Job drawing, mm, ordinate dimensions from the low corner. One solid piece. Round coordinates to 2 decimals unless told otherwise and drop trailing zeros. Loops run counter-clockwise (first coordinate to the right, second up) from the corner with the lowest first, then second, coordinate; pieces in that order, holes last. Notation, with made-up numbers: M 22.5,83 L 43.5,83 A14 ccw 43.5,110 Z; hole C 31,14.5 d3. An arc over 180 degrees is marked long. Put each result on its own line as item: value. Start each with the question number.
1) Slice it at C-C on z = 20. Give the cut face in (x, y).
2) Slice it at A-A on z = 49. Give the cut face in (x, y), then the cut area to 3 significant figures.
3) Probe line 1 along Z through (x, y) = (50, 4.5); line 2 along Z through (x, y) = (27.5, 4.6). List the from-to ranges inside material, lowest first.
4) Slice it at D-D on x = 49. Give the cut face in (y, z).
5) Drop flat-ended pins along their axis: pin 1 Ø1.5 at (y, z) = (2, 45) entering from -X; pin 2 Ø1.5 at (x, y) = (34, 3.5) entering from -Z. Give the stop position or say it passes through.
6) Slice it at B-B on x = 31. Give the cut face in (y, z).
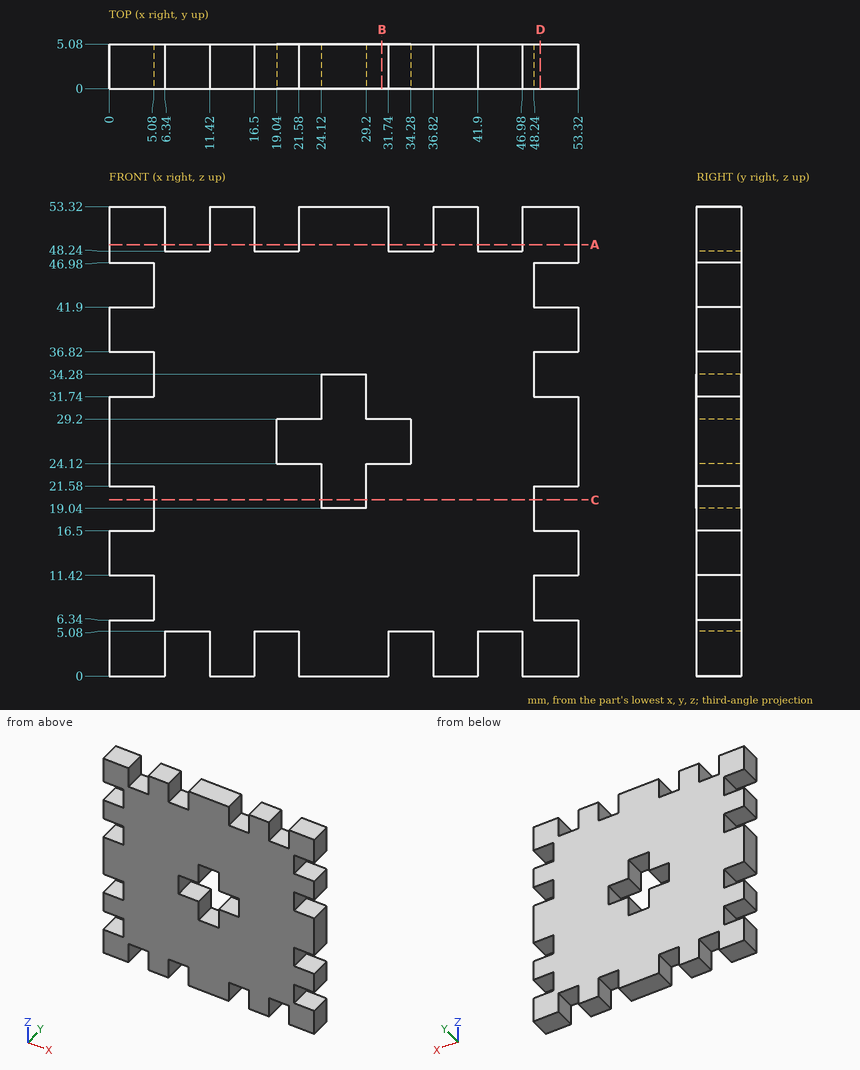
Recorded:
1. outline: M 5.08,0 L 24.12,0 L 24.12,5.08 L 5.08,5.08 Z; M 29.2,0 L 48.24,0 L 48.24,5.08 L 29.2,5.08 Z
2. outline: M 0,0 L 6.34,0 L 6.34,5.08 L 0,5.08 Z; M 11.42,0 L 16.5,0 L 16.5,5.08 L 11.42,5.08 Z; M 21.58,0 L 31.74,0 L 31.74,5.08 L 21.58,5.08 Z; M 36.82,0 L 41.9,0 L 41.9,5.08 L 36.82,5.08 Z; M 46.98,0 L 53.32,0 L 53.32,5.08 L 46.98,5.08 Z
2. area: 168 mm2
3. line 1: z = 0 to 6.34, 11.42 to 16.5, 21.58 to 31.74, 36.82 to 41.9, 46.98 to 53.32
3. line 2: z = 0 to 19.04, 34.28 to 53.32
4. outline: M 0,0 L 5.08,0 L 5.08,6.34 L 0,6.34 Z; M 0,11.42 L 5.08,11.42 L 5.08,16.5 L 0,16.5 Z; M 0,21.58 L 5.08,21.58 L 5.08,31.74 L 0,31.74 Z; M 0,36.82 L 5.08,36.82 L 5.08,41.9 L 0,41.9 Z; M 0,46.98 L 5.08,46.98 L 5.08,53.32 L 0,53.32 Z
5. pin 1: stops at x = 5.08
5. pin 2: stops at z = 5.08
6. outline: M 0,0 L 5.08,0 L 5.08,24.12 L 0,24.12 Z; M 0,29.2 L 5.08,29.2 L 5.08,53.32 L 0,53.32 Z
